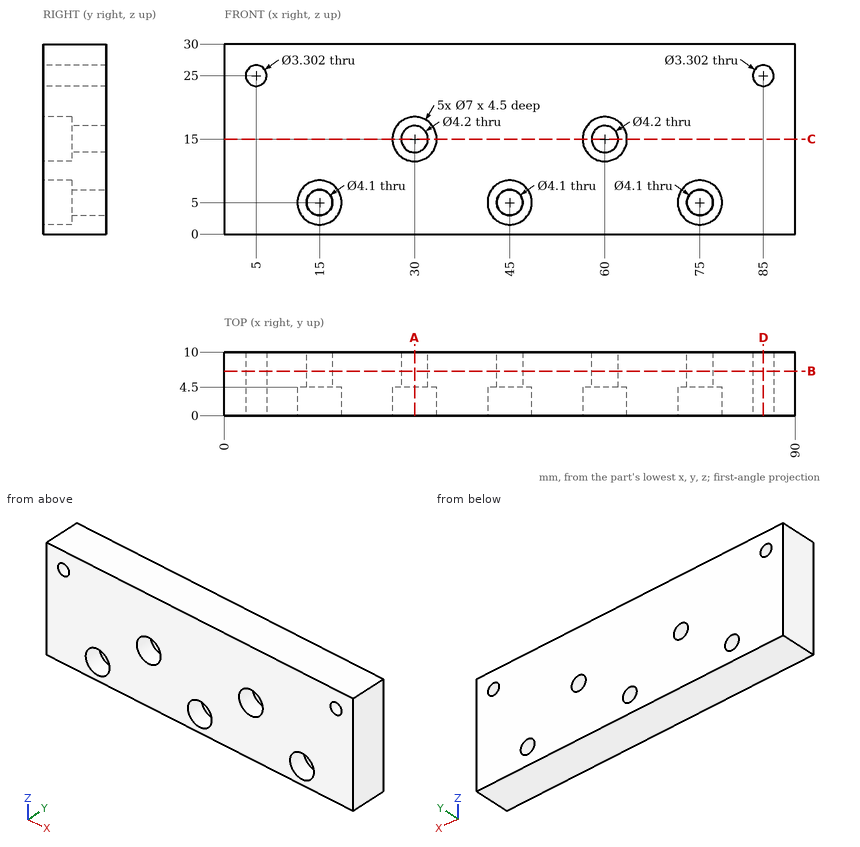
The figure shows three views and two pictorial views of one solid part (mm, origin at its lowest corner). Answer the questions. Give positions to 0.01 mm unless a question says otherwise; leave off trailing zeros. Write each loop counter-clockwise with the first axis right and the second up, starting at its lowest first coordinate (ties: lowest second). Pieces come first, ordered by that corner, then holes. Notation, with made-up numbers: (2, 22.5) -> (24, 22.5) arc R22 ccw to (24, 45.5) -> close; hole circle Ø6 at (50, 70). An arc over 180 degrees is marked (long way). Write each question's results on one line, items separated by ' | '.
1. Find section A-A on x = 30. Determine the outline of the cut face in (y, z).
Data:
outline: (0, 0) -> (10, 0) -> (10, 12.9) -> (4.5, 12.9) -> (4.5, 11.5) -> (0, 11.5) -> close; (0, 18.5) -> (4.5, 18.5) -> (4.5, 17.1) -> (10, 17.1) -> (10, 30) -> (0, 30) -> close
2. Find section B-B on y = 7. Determine the outline of the cut face in (x, z).
Data:
outline: (0, 0) -> (90, 0) -> (90, 30) -> (0, 30) -> close; hole circle Ø3.3 at (5, 25); hole circle Ø4.1 at (15, 5); hole circle Ø4.2 at (30, 15); hole circle Ø4.1 at (45, 5); hole circle Ø4.2 at (60, 15); hole circle Ø4.1 at (75, 5); hole circle Ø3.3 at (85, 25)
3. Find section C-C on z = 15. Determine the outline of the cut face in (x, y).
Data:
outline: (0, 0) -> (26.5, 0) -> (26.5, 4.5) -> (27.9, 4.5) -> (27.9, 10) -> (0, 10) -> close; (32.1, 4.5) -> (33.5, 4.5) -> (33.5, 0) -> (56.5, 0) -> (56.5, 4.5) -> (57.9, 4.5) -> (57.9, 10) -> (32.1, 10) -> close; (62.1, 4.5) -> (63.5, 4.5) -> (63.5, 0) -> (90, 0) -> (90, 10) -> (62.1, 10) -> close
4. Straight lines are drawn through the part: L1, parallel to X at y = 6.3, z = 5; L2, parallel to X at y = 1.75, z = 25.25; L3, parallel to Z at x = 30, y = 6.2. For each, find the intervals that lie inside material, in ascending order.
Data:
L1: 0 to 12.95, 17.05 to 42.95, 47.05 to 72.95, 77.05 to 90 | L2: 0 to 3.37, 6.63 to 83.37, 86.63 to 90 | L3: 0 to 12.9, 17.1 to 30
5. This flat-tipped pin is pushed along its axis until it touches: pin 1 Ø5.5 at (x, z) = (60, 15) entering from -Y. Where does it stop, or does it pass through?
Data:
pin 1: y = 4.5
6. Find section D-D on x = 85. Determine the outline of the cut face in (y, z).
Data:
outline: (0, 0) -> (10, 0) -> (10, 23.35) -> (0, 23.35) -> close; (0, 26.65) -> (10, 26.65) -> (10, 30) -> (0, 30) -> close
